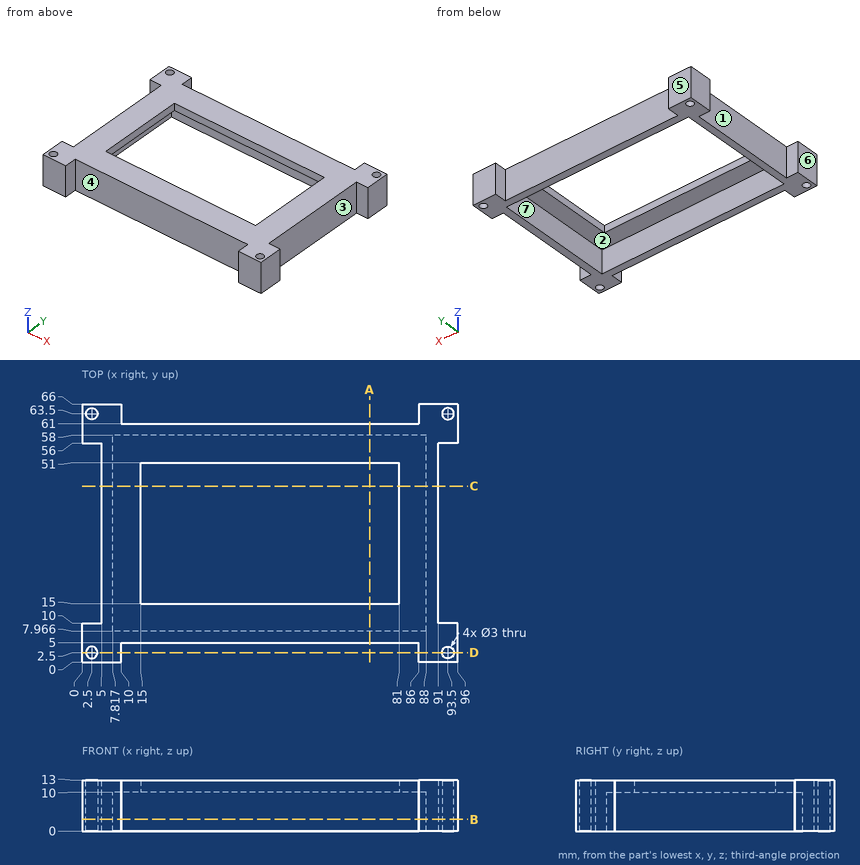
Input: dimensioned drawing with shaded views. Units: mm. Origin: part minimum x, y, z. A direction names the side the tool comes from. Round coordinates to 2 decimals unless told otherwise and drop trailing zeros. Loops run counter-clockwise (first coordinate to the right, second up) from the corner with the lowest first, then second, coordinate; pieces in that order, holes last. Notation, with made-up numbers: M 89,38.25 L 121,38.25 A20 ccw 121,43.25 Z; hole C -17,9.25 d8. An arc over 180 degrees is marked long. Answer in a Markdown table with one row per item. Add a question column.
1. Section D-D (y = 2.5). Output: boundary loops of the cut face in (x, z).
2. Ray query, probe 1 along Y at (x, z) = (93.5, 9.75); probe 2 along Y at (x, z) = (55, 6.25); probe 3 along Y at (x, z) = (52, 12.5). Return the intervals inside material, ascending.
3. Set-up query: the marked faces 1, 2, 3 and 4. Return all of +Z, -Z, +X, -X, +Y, -Y with unobstructed straight access to the full face (end or side cutting, diameter ignored); none if empty.
4. Section B-B (z = 3). Output: boundary loops of the cut face in (x, y), and give its area (3 significant figures).
5. Section A-A (x = 73.5). Output: boundary loops of the cut face in (y, z).
6. Section C-C (y = 45). Output: boundary loops of the cut face in (x, z), and give its area (3 significant figures).
7. Mould query, pull axis Y, two halves, no side actions, for the marked faces 5, 6 and 7. Classes: released by +Y, released by -Y, zero draft, split by the parting line, or undercut.
8. Contact query for flat-ended pins moving along their axis: pin 1 (6 mm diameter, centred on y = 26, z = 2.5, fed in from +X); pin 2 (5 mm diameter, centred on x = 77.5, z = 4, fed in from +Y); pin 3 (4 mm diameter, centred on x = 22, y = 15, fed in from -Z). Output: stop coordinate, or through.
Values follow:
| question | item | result |
|---|---|---|
| 1 | outline | M 0,0 L 1,0 L 1,13 L 0,13 Z; M 4,0 L 10,0 L 10,13 L 4,13 Z; M 86,0 L 92,0 L 92,13 L 86,13 Z; M 95,0 L 96,0 L 96,13 L 95,13 Z |
| 2 | probe 1 | 0 to 1, 4 to 10, 56 to 62, 65 to 66 |
| 2 | probe 2 | 5 to 7.97, 58 to 61 |
| 2 | probe 3 | 5 to 15, 51 to 61 |
| 3 | face 1 | +Z, -Z, -X |
| 3 | face 2 | -Z |
| 3 | face 3 | +Z, -Z, +X |
| 3 | face 4 | +Z, -Z, -Y |
| 4 | outline | M 0,0 L 10,0 L 10,5 L 86,5 L 86,0 L 96,0 L 96,10 L 91,10 L 91,56 L 96,56 L 96,66 L 86,66 L 86,61 L 10,61 L 10,66 L 0,66 L 0,56 L 5,56 L 5,10 L 0,10 Z; hole C 2.5,2.5 d3; hole C 2.5,63.5 d3; hole M 7.82,7.97 L 88,7.97 L 88,58 L 7.82,58 Z; hole C 93.5,2.5 d3; hole C 93.5,63.5 d3 |
| 4 | area | 1,080 mm^2 |
| 5 | outline | M 5,0 L 7.97,0 L 7.97,10 L 15,10 L 15,13 L 5,13 Z; M 51,10 L 58,10 L 58,0 L 61,0 L 61,13 L 51,13 Z |
| 6 | outline | M 5,0 L 7.82,0 L 7.82,10 L 15,10 L 15,13 L 5,13 Z; M 81,10 L 88,10 L 88,0 L 91,0 L 91,13 L 81,13 Z |
| 6 | area | 118 mm^2 |
| 7 | face 5 | released by +Y |
| 7 | face 6 | zero draft |
| 7 | face 7 | undercut |
| 8 | pin 1 | x = 91 |
| 8 | pin 2 | y = 61 |
| 8 | pin 3 | z = 10 |
